Autodesk Inventor part; units mm, degrees
ref_plane "YZ Plane" through (0, 0, 0) normal (1, 0, 0) x (0, 1, 0)
ref_plane "XZ Plane" through (0, 0, 0) normal (0, 1, 0) x (-1, 0, 0)
ref_plane "XY Plane" through (0, 0, 0) normal (0, 0, 1) x (1, 0, 0)
sketch "Sketch1" plane through (0, 0, 0) normal (1, 0, 0) x (0, 1, 0)
  line L0 (0, 0) -> (203.2, 0) construction
  line L1 (203.2, 0) -> (203.2, 25.4) construction
  line L2 (203.2, 25.4) -> (0, 25.4) construction
  line L3 (0, 25.4) -> (0, 0) construction
  line L4 (0, 0) -> (25.4, 0) construction
  line L5 (25.4, 0) -> (25.4, -609.6) construction
  line L6 (25.4, -609.6) -> (0, -609.6) construction
  line L7 (0, -609.6) -> (0, 0) construction
  circle A0 centre (14.2875, -23.8125) radius 11.1125 construction
  line L8 (-1.5875, -12.7) -> (150.8125, -12.7) construction
  line L9 (114.3, -12.7) -> (25.4, -12.7) construction
  line L10 (25.4, -12.7) -> (25.4, -419.1) construction
  line L11 (25.4, -419.1) -> (114.3, -419.1) construction
  line L12 (114.3, -419.1) -> (114.3, -12.7) construction
  circle A1 centre (14.2875, -23.8125) radius 7.9375 construction
  circle A2 centre (14.2875, -23.8125) radius 3.175
  circle A3 centre (12.7, -114.3) radius 3.9688
  circle A4 centre (12.7, -241.3) radius 3.9688
  circle A5 centre (12.7, -368.3) radius 3.9688
  circle A6 centre (12.7, -495.3) radius 3.9688 construction
  circle A7 centre (14.2875, -87.3125) radius 3.175
  circle A8 centre (14.2875, -87.3125) radius 11.1125 construction
  circle A9 centre (14.2875, -150.8125) radius 3.175
  circle A10 centre (14.2875, -150.8125) radius 11.1125 construction
  circle A11 centre (14.2875, -214.3125) radius 3.175
  circle A12 centre (14.2875, -214.3125) radius 11.1125 construction
  circle A13 centre (14.2875, -277.8125) radius 3.175
  circle A14 centre (14.2875, -277.8125) radius 11.1125 construction
  circle A15 centre (14.2875, -341.3125) radius 3.175
  circle A16 centre (14.2875, -341.3125) radius 11.1125 construction
  circle A17 centre (14.2875, -404.8125) radius 3.175
  circle A18 centre (14.2875, -404.8125) radius 11.1125 construction
  line L13 (0, -2.4888) -> (22.225, -2.4888)
  line L14 (22.225, -2.4888) -> (22.225, -428.625)
  line L15 (22.225, -428.625) -> (0, -428.625)
  line L16 (0, -428.625) -> (0, -2.4888)
  dimension "d0" = 203.2
  dimension "d1" = 25.4
  dimension "d2" = 25.4
  dimension "d3" = 609.6
  dimension "d4" = 12.7
  dimension "d6" = 22.225
  dimension "d7" = 406.4
  dimension "d8" = 88.9
  dimension "d10" = 15.875
  dimension "d11" = 6.35
  dimension "d12" = 7.9375
  dimension "d13" = 12.7
  dimension "d14" = 114.3
  dimension "d17" = 127
  dimension "d24" = 63.5
  dimension "d29" = 22.225
extrude "Extrusion1" add sketch "Sketch1" along normal blind 2.3876
sketch "Sketch2" plane through (0, 0, -2.4888) normal (0, 0, 1) x (1, 0, 0)
  line L0 (0, 0) -> (-19.8374, 0)
  line L1 (-19.8374, 0) -> (-19.8374, 2.3876)
  line L2 (-19.8374, 2.3876) -> (0, 2.3876)
  line L3 (0, 2.3876) -> (0, 0)
  dimension "d32" = 19.8374
  dimension "d33" = 2.3876
extrude "Extrusion2" add sketch "Sketch2" against normal up to surface (426.1362 mm away)
sketch "Sketch3" plane through (-19.8374, 2.3876, -2.4888) normal (0, 1, 0) x (1, 0, 0)
  circle A0 centre (9.9187, 25.4) radius 3.175
  line L0 (19.8374, 0) -> (0, 0)
  line L1 (9.9187, 0) -> (9.9187, 25.4) construction
  circle A1 centre (9.9187, 400.7362) radius 3.175
  line L2 (19.8374, 426.1362) -> (0, 426.1362) construction
  point P0 (19.8374, -2.4888)
  dimension "d36" = 6.35
  dimension "d37" = 25.4
  dimension "d38" = 6.35
  dimension "d39" = 25.4
extrude "Extrusion3" cut sketch "Sketch3" against normal through all
properties part number "BatteryDrawer_AngleBrackets"
Geometry check sheet. Reference: the model listing, model coordinates, mm. A direction names the side the tool comes from. Give positions to 0.01 mm unless a question says otherwise; leave off trailing zeros. Order: outer loops, then holes, each group sorted by start corner. A loop starts at its lowest first (then second) coordinate and runs counter-clockwise, first axis right, second up. Notation, with made-up numbers: (55.5, -9.75) - (79.5, -9.75) arc R18 ccw to (79.5, 7.25) - close; hole circle Ø1 at (-1, 21). An arc over 180 degrees is marked (long way). Use one line per item in the form item = value.
1) Depth check by flat-ended pin: pin 1 Ø6 at (x, y) = (-13.5, 6) entering from -Z; pin 2 Ø7.5 at (x, z) = (-9.92, -403.22) entering from +Y; pin 3 Ø10.5 at (y, z) = (12.7, -114.3) entering from -X. Enter the tip coordinate at first touch or a pass-through.
Working result:
pin_1 = through
pin_2 = 2.39
pin_3 = 0
2) Sectioned sample at A-A (z = -114.3). Record the boundary of the cut face in (x, y) (3 decimals), and give its area (3 significant figures).
Working result:
outline = (-19.837, 0) - (2.388, 0) - (2.388, 8.731) - (0, 8.731) - (0, 2.388) - (-19.837, 2.388) - close; (0, 16.669) - (2.388, 16.669) - (2.388, 22.225) - (0, 22.225) - close
area = 81.5 mm^2
3) Sectioned sample at B-B (z = -64). Record the boundary of the cut face in (x, y) (3 decimals).
Working result:
outline = (-19.837, 0) - (2.388, 0) - (2.388, 22.225) - (0, 22.225) - (0, 2.388) - (-19.837, 2.388) - close
4) Access from +Z, -Z, +X, -X, +Y, -Y to the whole of each face (thin tool, end or side, straight path). Record for faces 4 (the face through (0, 10, -213)), 5 (the face through (1.18, 14.83, -371.65)).
Working result:
face_4 = +Z, -Z, -X, +Y
face_5 = +X, -X
5) Draft check along Y on faces 1 (the face through (1.177, 16.366, -112.78)), 2 (the face through (2.388, 11, -213)), 3 (the face through (-10, 2.388, -213)). Enter one of: released by +Y, released by -Y, zero draft, split by the parting line, or undercut.
Working result:
face_1 = undercut
face_2 = zero draft
face_3 = released by +Y
6) Material ranges on probe 1 along Y at (x, z) = (-10.5, -44), recorded low to high. Write a range as from..to.
Working result:
probe_1 = 0..2.39
